Read the model definition and answer for the solid it produces. Units are mm, in the model's axes. Face numbers are marked on the shaded views. A direction names the side the tool comes from. Coordinates: 2 decimals unless noted, no trailing zeros. Loops run counter-clockwise (first coordinate to the right, second up) from the corner with the lowest first, then second, coordinate; pieces in that order, holes last. Notation, with made-up numbers: (68.25, 6) -> (84.25, 6) arc R24 ccw to (84.25, 19) -> close; hole circle Ø10 at (76.5, 41.25). An arc over 180 degrees is marked (long way). Answer as CSV lines item,"result".
```python
from build123d import *

# Parameters (mm, degrees)
Y_KSEKLIK_EKSTR_ZYON1_DEPTH = 10
IZIM2_W                     = 120
IZIM2_H                     = 1
Y_KSEKLIK_EKSTR_ZYON2_DEPTH = 3
IZIM4_W                     = 2
IZIM4_H                     = 10
Y_KSEKLIK_EKSTR_ZYON3_DEPTH = 4


with BuildPart() as part:
    # Çizim1 → Yükseklik-Ekstrüzyon1 (new body)
    with BuildSketch(Plane.XY):
        Polygon((0, 0), (-120, 0), (-120, -1), (2, -1), (2, 3), (0, 3), align=None)
    extrude(amount=Y_KSEKLIK_EKSTR_ZYON1_DEPTH)

    # Çizim2 → Yükseklik-Ekstrüzyon2 (add)
    with BuildSketch(Plane(origin=(0, 0, 0), x_dir=(1, 0, 0), z_dir=(0, 1, 0))):
        with Locations((-60, -9.5)):
            Rectangle(IZIM2_W, IZIM2_H)
    extrude(amount=Y_KSEKLIK_EKSTR_ZYON2_DEPTH)

    # Çizim4 → Yükseklik-Ekstrüzyon3 (add)
    with BuildSketch(Plane(origin=(0, 3, 0), x_dir=(1, 0, 0), z_dir=(0, 1, 0))):
        with Locations((1, -5)):
            Rectangle(IZIM4_W, IZIM4_H)
    extrude(amount=Y_KSEKLIK_EKSTR_ZYON3_DEPTH)


solid = part.part
```
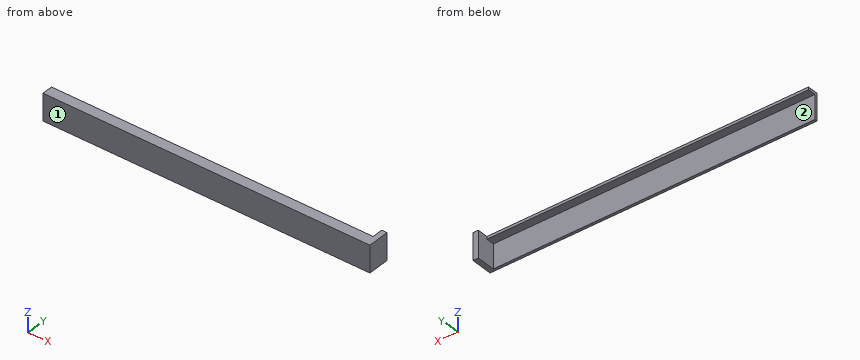
Q1. A cutting plane is placed at A-A, the plane z = 2.25. Write down the section's boundary in (x, y), and give its area (3 significant figures).
Results:
outline,"(-120, -1) -> (2, -1) -> (2, 7) -> (0, 7) -> (0, 0) -> (-120, 0) -> close"
area,"136 mm²"
Q2. Given pin 1 Ø1.5 at (y, z) = (0.5, 2) entering from -X; pin 2 Ø1.5 at (x, y) = (-50, 5.5) entering from -Z; pin 3 Ø1 at (x, y) = (-82, 2.5) entering from -Z; pin 4 Ø1.1 at (x, z) = (-86, 9.5) entering from +Y, each flat-ended and moving along its own axis, determine where each tip first touches the part or whether it passes through.
Results:
pin 1,"stops at x = -120"
pin 2,"passes through"
pin 3,"stops at z = 9"
pin 4,"stops at y = 3"
Q3. A cutting plane is placed at B-B, the plane x = -49. Write down the section's boundary in (y, z).
Results:
outline,"(-1, 0) -> (0, 0) -> (0, 9) -> (3, 9) -> (3, 10) -> (-1, 10) -> close"
Q4. For the marked faces 1 and 2, determine the directions among +Z, -Z, +X, -X, +Y, -Y from which every point of the face is accessible in a straight line to the end or side of a thin tool.
Results:
face 1,"+Z, -Z, +X, -X, -Y"
face 2,"-Z, -X, +Y"
Q5. Find the intervals of material crossed by probe 1 along Z at (x, y) = (-74, 1); probe 2 along X at (y, z) = (2, 6.25); probe 3 along Y at (x, z) = (-103, 4.5), in increasing order. Write a range as [from, to].
Results:
probe 1,"z = [9, 10]"
probe 2,"x = [0, 2]"
probe 3,"y = [-1, 0]"
Q6. A cutting plane is placed at C-C, the plane y = 5.5. Write down the section's boundary in (x, z).
Results:
outline,"(0, 0) -> (2, 0) -> (2, 10) -> (0, 10) -> close"
